```python
from build123d import *


with BuildPart() as f1:
    # F0 (on Front) → F1 (revolve)
    with BuildSketch(Plane.XZ):
        with BuildLine():
            Line((0, 80), (0, 0))
            Line((0, 0), (3, 0))
            Line((3, 0), (3, 49))
            ThreePointArc((3, 49), (3.292893, 49.707107), (4, 50))
            Line((4, 50), (5, 50))
            Line((5, 50), (5, 79))
            ThreePointArc((5, 79), (4.707107, 79.707107), (4, 80))
            Line((4, 80), (0, 80))
        make_face()
    revolve(axis=Axis((0, 0, 40), (0, 0, 1)))


solid = f1.part
```
Could you check a few things on this model? Use its own coordinates, in mm. A direction names the side the tool comes from. Round coordinates to 2 decimals unless told otherwise and drop trailing zeros. Order: outer loops, then holes, each group sorted by start corner. A loop starts at its lowest first (then second) coordinate and runs counter-clockwise, first axis right, second up. Notation, with made-up numbers: M -36.5,-8.5 L -31.5,-8.5 A22 ccw -31.5,1.5 Z; hole C -30.5,4 d10. An arc over 180 degrees is marked long. One line per question, with ' | ' between items. Start each with the question number.
(1) For P1, Ø5, axis at x = 3, z = 17.5, coming from the -Y side; P2, Ø4, axis at y = -1, z = 32, coming from the -X side; P3, Ø1.5, axis at y = 2.5, z = 42, coming from the -X side; P4, Ø4, axis at x = -4, y = 1.5, coming from the +Z side, each with a flat end and sliding along its axis, tell me the tip position at first contact or that it passes through.
(2) Suppose I cut it at A-A on y = 0. List the corners of the cut face in (x, z) for me, then the cut area to 3 significant figures.
(3) Please list where these lines run through material, in increasing order: line 1 along Y through (x, z) = (3, 74); line 2 along Y through (x, z) = (4, 59); line 3 along X through (y, z) = (-2.5, 70).
(4) Suppose I cut it at C-C on z = 53.5. List the corners of the cut face in (x, y) for me.
(5) For faces 1 (the face through (-3, 0, 25)), 2 (the face through (-1.08, -4.88, 64.7)), which set-ups out of +Z, -Z, +X, -X, +Y, -Y let a thin tool reach every point of the face, with its end or its side?
Geometry results:
1) P1: y = -2.96 | P2: x = -3 | P3: x = -2.44 | P4: z = 80
2) outline: M -5,50 L -4,50 A1 cw -3,49 L -3,0 L 3,0 L 3,49 A1 cw 4,50 L 5,50 L 5,79 A1 ccw 4,80 L -4,80 A1 ccw -5,79 Z | area: 600 mm²
3) line 1: -4 to 4 | line 2: -3 to 3 | line 3: -4.33 to 4.33
4) outline: C 0,0 d10
5) face 1: -Z | face 2: +Z, -Z
